Work out the finished part from the listing and answer in its coordinate system (mm). A direction names the side the tool comes from. Coordinates: 2 decimals unless noted, no trailing zeros. Loops run counter-clockwise (first coordinate to the right, second up) from the corner with the lowest first, then second, coordinate; pieces in that order, holes last. Notation, with made-up numbers: (67, 28) -> (112, 28) arc R21 cw to (112, 47) -> close; hole circle Ø10 at (24.25, 22.5). An arc over 180 degrees is marked (long way). Use a Markdown table: item, result.
from build123d import *

# Parameters (mm, degrees)
BOSS_EXTRUDE1_DEPTH     = 1346.2
CUT_EXTRUDE1_DEPTH      = 279.4
CUT_EXTRUDE2_DEPTH      = 1441.932396055
CUT_EXTRUDE2_DEPTH_BACK = 279.4
SKETCH5_W               = 660.4
SKETCH5_H               = 424.18
BOSS_EXTRUDE2_DEPTH     = 177.8
SKETCH6_W               = 660.4
SKETCH6_H               = 424.18
BOSS_EXTRUDE3_DEPTH     = 177.8
SKETCH7_W               = 431.8
SKETCH7_H               = 431.8
CUT_EXTRUDE3_DEPTH      = 660.4


with BuildPart() as part:
    # Sketch1 → Boss-Extrude1 (new body)
    with BuildSketch(Plane(origin=(0, 0, 0), x_dir=(0, 0, -1), z_dir=(1, 0, 0))):
        Polygon((100.623076923, 266.7), (-330.2, -266.7), (330.2, -266.7), (330.2, 266.7), (203.2, 266.7), align=None)
        Polygon((203.2, 393.7), (100.623076923, 266.7), (203.2, 266.7), (330.2, 266.7), (330.2, 393.7), align=None)
    extrude(amount=BOSS_EXTRUDE1_DEPTH)

    # Sketch2 → Cut-Extrude1 (cut)
    with BuildSketch(Plane(origin=(1346.2, 0, 0), x_dir=(0, 0, -1), z_dir=(1, 0, 0))):
        Polygon((330.2, 393.7), (330.2, 266.7), (100.623076923, 266.7), (203.2, 393.7), align=None)
    extrude(amount=-CUT_EXTRUDE1_DEPTH, mode=Mode.SUBTRACT)

    # Sketch3 → Cut-Extrude2 (cut, two sides: drawn at the far end of the back side and taken through both)
    with BuildSketch(Plane.ZY.offset(-CUT_EXTRUDE2_DEPTH_BACK)):
        Polygon((-330.2, 2271.593273182), (-330.2, 393.7), (-330.2, 266.7), (-100.623076923, 266.7), (1777.270196259, 266.7), (4365.963516587, 2987.839370769), (2258.493320327, 4992.732643951), align=None)
    extrude(amount=CUT_EXTRUDE2_DEPTH + CUT_EXTRUDE2_DEPTH_BACK, mode=Mode.SUBTRACT)

    # Sketch5 → Boss-Extrude2 (add)
    with BuildSketch(Plane(origin=(1346.2, 0, 0), x_dir=(0, 0, -1), z_dir=(1, 0, 0))):
        with Locations((0, -54.61)):
            Rectangle(SKETCH5_W, SKETCH5_H)
    extrude(amount=-BOSS_EXTRUDE2_DEPTH)

    # Sketch6 → Boss-Extrude3 (add)
    with BuildSketch(Plane.ZY):
        with Locations((0, -54.61)):
            Rectangle(SKETCH6_W, SKETCH6_H)
    extrude(amount=-BOSS_EXTRUDE3_DEPTH)

    # Sketch7 → Cut-Extrude3 (cut)
    with BuildSketch(Plane(origin=(0, 56.109668756, 69.469113697), x_dir=(1, 0, 0), z_dir=(0, 0.6283371070876211, 0.7779411802037217))):
        with Locations((681.021503016, -66.438627043)):
            Rectangle(SKETCH7_W, SKETCH7_H)
    extrude(amount=-CUT_EXTRUDE3_DEPTH, mode=Mode.SUBTRACT)


solid = part.part
Q1. Section D-D on x = 1104 is taken. Determine the outline of the cut face in (y, z).
Solved:
| item | result |
|---|---|
| outline | (-266.7, -330.2) -> (266.7, -330.2) -> (266.7, -100.62) -> (-266.7, 330.2) -> close |
Q2. Given pin 1 Ø4 at (x, z) = (919.5, -38.5) entering from +Y; pin 2 Ø12 at (y, z) = (145.5, 209.5) entering from -X; pin 3 Ø8 at (x, z) = (236, 48) entering from +Y, each flat-ended and moving along its own axis, determine where each tip first touches the part or whether it passes through.
Solved:
| item | result |
|---|---|
| pin 1 | y = 192.26 |
| pin 2 | x = 0 |
| pin 3 | y = 87.64 |
Q3. Determine the mould class of faces 5 (the flat face through (0, -56, 5)), 6 (the flat face through (896.922, -84, -70)), 7 (the flat face through (88, -58, 330.2)) for opening direction X: pulls with the +X half, pulls with the -X half, needs draft (parallel to the pull), parting line crosses it, or undercut.
Solved:
| item | result |
|---|---|
| face 5 | pulls with the -X half |
| face 6 | undercut |
| face 7 | needs draft |
Q4. Section C-C on z = 199.5 is taken. Determine the outline of the cut face in (x, y), and give its area (3 significant figures).
Solved:
| item | result |
|---|---|
| outline | (0, -266.7) -> (1346.2, -266.7) -> (1346.2, 157.48) -> (1168.4, 157.48) -> (1168.4, -104.88) -> (896.92, -104.88) -> (896.92, -201.8) -> (465.12, -201.8) -> (465.12, -104.88) -> (177.8, -104.88) -> (177.8, 157.48) -> (0, 157.48) -> close |
| area | 269,000 mm² |
Q5. For faces 1 (the flat face through (88, 157.48, 156)), 2 (the flat face through (677.999, -214.394, 183.902)), 3 (the flat face through (1066.8, 331, -243)), 4 (the flat face through (279.4, 331, -243)), determine the directions among +Z, -Z, +X, -X, +Y, -Y from which every point of the face is accessible in a straight line to the end or side of a thin tool.
Solved:
| item | result |
|---|---|
| face 1 | +Z, +X, -X, +Y |
| face 2 | -Z, +Y |
| face 3 | +Z, -Z, +X, +Y |
| face 4 | +Z, -Z, -X, +Y |
Q6. Section B-B on y = -118 is taken. Determine the outline of the cut face in (x, z).
Solved:
| item | result |
|---|---|
| outline | (0, -330.2) -> (465.12, -330.2) -> (465.12, 210.1) -> (177.8, 210.1) -> (177.8, 330.2) -> (0, 330.2) -> close; (896.92, -330.2) -> (1346.2, -330.2) -> (1346.2, 330.2) -> (1168.4, 330.2) -> (1168.4, 210.1) -> (896.92, 210.1) -> close |
Q7. Consider line 1 (X direction, y = -100, z = 221.5); line 2 (X direction, y = -158.5, z = -304); line 3 (Y direction, x = 1257, z = -200). Determine where each line is inside the solid, lowest interval first. Write a range as [from, to].
Solved:
| item | result |
|---|---|
| line 1 | [0, 177.8], [1168.4, 1346.2] |
| line 2 | [0, 465.12], [896.92, 1346.2] |
| line 3 | [-266.7, 266.7] |
Q8. Section A-A on x = 759.5 is taken. Determine the outline of the cut face in (y, z), and give its area (3 significant figures).
Solved:
| item | result |
|---|---|
| outline | (-266.7, 119.14) -> (-163.53, 246.87) -> (-266.7, 330.2) -> close; (-74.58, -330.2) -> (393.7, -330.2) -> (393.7, -203.2) -> (172.38, -24.44) -> close |
| area | 96,500 mm² |
